from build123d import *

# Parameters (mm, degrees)
PAD014_DEPTH                        = 3
SKETCH055_R                         = 1.65
POCKET019_DEPTH                     = 364.282338
POCKET019_DEPTH_BACK                = 367.282338
BODY001003005003003_PLACEMENT_ANGLE = 60
CLONE001_PLACEMENT_ANGLE            = 140


with BuildPart() as part:
    # Sketch052 → Pad014 (new body)
    with BuildSketch(Plane.XY):
        with BuildLine():
            ThreePointArc((152.959511, 127.101705), (84.480895, 180.040089), (0, 198.875477))
            Line((0, 198.875477), (0, 208.875477))
            ThreePointArc((160.650731, 133.492724), (88.728824, 189.092995), (0, 208.875477))
            ThreePointArc((152.959511, 127.101705), (160.000631, 126.451604), (160.650731, 133.492724))
        make_face()
    pad014 = extrude(amount=PAD014_DEPTH)

    # Sketch055 → Pocket019 (cut, two sides)
    with BuildSketch(Plane.XY) as pocket019_sk:
        with Locations((143.11, 145.205847)):
            Circle(SKETCH055_R)
        with BuildLine():
            Line((0, 202.225477), (0, 205.525477))
            ThreePointArc((0, 202.225477), (1.65, 203.875477), (0, 205.525477))
        make_face()
    pocket019 = extrude(amount=-POCKET019_DEPTH, mode=Mode.SUBTRACT) + extrude(pocket019_sk.sketch, amount=POCKET019_DEPTH_BACK, mode=Mode.SUBTRACT)

    # Mirrored019: Pad014, Pocket019 across Sketch052 V_Axis
    add(pad014.mirror(Plane(origin=(0, 0, 0), x_dir=(0, 0, 1), z_dir=(1, 0, 0))))
    add(pocket019.mirror(Plane(origin=(0, 0, 0), x_dir=(0, 0, 1), z_dir=(1, 0, 0))), mode=Mode.SUBTRACT)


with BuildPart() as part_1:
    # Body001003005003003 placement: moved
    add(part.part.rotate(Axis((0, 0, 0), (0, 0, 1)), BODY001003005003003_PLACEMENT_ANGLE))


with BuildPart() as part_2:
    # Clone001 placement: moved
    add(part_1.part.moved(Location((1303, 744, 0))).rotate(Axis((1303, 744, 0), (0, 0, 1)), CLONE001_PLACEMENT_ANGLE))


solid = part_2.part
Check sheet for the modelled part. Datum: model origin and axes. Units: mm. Round coordinates to 2 decimals unless told otherwise and drop trailing zeros. Order: outer loops, then holes, each group sorted by start corner. A loop starts at its lowest first (then second) coordinate and runs counter-clockwise, first axis right, second up.
(1) Cross-section at A-A, the plane z = 1.75. Enter the section's corners in (x, y).
(2) Go/stop test with flat-tipped pins: P1, Ø1.5, axis at y = 632, z = 2, coming from the +X side; P2, Ø2, axis at x = 1372.73, y = 552.42, coming from the +Z side (3 decimals); P3, Ø1.5, axis at x = 1375, z = 2.5, coming from the +Y side. Record where each tip stops, or that it passes through.
(3) Scan lines: probe 1 along X at (y, z) = (560.5, 0.5); probe 2 along X at (y, z) = (562.5, 2.55); probe 3 along X at (y, z) = (573.5, 2.35). Record each from-to range of solid material in increasing order.
(4) Cross-section at C-C, the plane x = 1261. Enter the section's corners in (y, z), and give its area (3 significant figures).
(5) Cross-section at B-B, the plane y = 667. Enter the section's corners in (x, z), and give its area (3 significant figures).
Check sheet entries:
1. outline: (1197.69, 563.61) arc R208.88 ccw to (1374.44, 547.72) arc R208.88 ccw to (1499.62, 673.5) arc R5 ccw to (1490.21, 676.88) arc R198.88 cw to (1371.02, 557.12) arc R198.88 cw to (1202.74, 572.25) arc R5 ccw to start; hole circle Ø3.3 at (1218.18, 558.6); hole circle Ø3.3 at (1372.73, 552.42); hole circle Ø3.3 at (1487.14, 656.5)
2. P1: stops at x = 1479.78
2. P2: passes through
2. P3: stops at y = 558.91
3. probe 1: x = 1203.22 to 1226.32, 1379.68 to 1402.78
3. probe 2: x = 1199.62 to 1221.7, 1384.3 to 1406.38
3. probe 3: x = 1405.38 to 1423.66
4. outline: (539.39, 0) - (549.61, 0) - (549.61, 3) - (539.39, 3) - close
4. area: 30.7 mm2
5. outline: (1486.36, 0) - (1497.16, 0) - (1497.16, 3) - (1486.36, 3) - close
5. area: 32.4 mm2
